from build123d import *

# Parameters (mm, degrees)
BOSS_EXTRUDE1_DEPTH = 0.2
BOSS_EXTRUDE2_DEPTH = 39
CUT_EXTRUDE1_DEPTH  = 10


with BuildPart() as part:
    # Sketch1 → Boss-Extrude1 (new body)
    with BuildSketch(Plane.XY):
        with BuildLine():
            Line((0, 0), (39, 0))
            Line((39, 0), (39, 7.5))
            ThreePointArc((39, 7.5), (37.881966011, 7.763932023), (37, 8.5))
            ThreePointArc((37, 8.5), (35.5, 10), (37, 11.5))
            ThreePointArc((37, 11.5), (37.881966011, 12.236067977), (39, 12.5))
            Line((39, 12.5), (39, 19.5))
            Line((39, 19.5), (0, 19.5))
            Line((0, 19.5), (0, 12.5))
            ThreePointArc((0, 12.5), (1.118033989, 12.236067977), (2, 11.5))
            ThreePointArc((2, 11.5), (3.5, 10), (2, 8.5))
            ThreePointArc((2, 8.5), (1.118033989, 7.763932023), (0, 7.5))
            Line((0, 7.5), (0, 0))
        make_face()
        with BuildLine():
            Line((21, 12.7), (21, 8.9))
            ThreePointArc((21, 8.9), (19.5, 7.4), (18, 8.9))
            Line((18, 8.9), (18, 12.7))
            ThreePointArc((18, 12.7), (19.5, 14.2), (21, 12.7))
        make_face(mode=Mode.SUBTRACT)
    extrude(amount=BOSS_EXTRUDE1_DEPTH)

    # Sketch2 → Boss-Extrude2 (add)
    with BuildSketch(Plane(origin=(39, 0, 0), x_dir=(0, 0, -1), z_dir=(1, 0, 0))):
        with BuildLine():
            Line((-0.7, 0.5), (-0.7, 6.5))
            Line((-0.7, 6.5), (-0.2, 6.5))
            Line((-0.2, 6.5), (-0.2, 0))
            Line((-0.2, 0), (0, 0))
            Line((0, 0), (0, 6.5))
            Line((0, 6.5), (0.5, 6.5))
            Line((0.5, 6.5), (0.5, 0.5))
            ThreePointArc((0.5, 0.5), (-0.1, -0.1), (-0.7, 0.5))
        make_face()
    extrude(amount=-BOSS_EXTRUDE2_DEPTH)

    # Sketch3 → Cut-Extrude1 (cut)
    with BuildSketch(Plane.XY.offset(0.2)):
        Polygon((17, 19.5), (19.5, 17.002927863), (22, 19.5), (22, 22.539691699), (17, 22.539691699), align=None)
    extrude(amount=-CUT_EXTRUDE1_DEPTH, mode=Mode.SUBTRACT)


solid = part.part
Work out the finished part from the listing and answer in its coordinate system (mm). A direction names the side the tool comes from. Give positions to 0.01 mm unless a question says otherwise; leave off trailing zeros. Write each loop counter-clockwise with the first axis right and the second up, starting at its lowest first coordinate (ties: lowest second). Pieces come first, ordered by that corner, then holes.
Q1. Straight lines are drawn through the part: L1, parallel to Z at x = 25, y = 9; L2, parallel to Y at x = 22.5, z = 0.05; L3, parallel to Y at x = 28, z = 0.55. For each, find the intervals that lie inside material, in ascending order.
Answer:
L1: z = 0 to 0.2
L2: y = -0.1 to 19.5
L3: y = 0.1 to 6.5
Q2. The part is cut by section B-B on x = 20.5. Give the vertices of the cut face in (y, z), and give its area (3 significant figures).
Answer:
outline: (0.5, -0.5) - (6.5, -0.5) - (6.5, 0) - (7.78, 0) - (7.78, 0.2) - (6.5, 0.2) - (6.5, 0.7) - (0.5, 0.7) arc R0.6 ccw to start; (13.82, 0) - (18, 0) - (18, 0.2) - (13.82, 0.2) - close
area: 8.86 mm2
Q3. Given pin 1 (2 mm diameter, centred on x = 13, y = 15.5, fed in from -Z); pin 2 (0.5 mm diameter, centred on x = 23.5, z = 0.5, fed in from +Y), each flat-ended and moving along its own axis, determine where each tip first touches the part or whether it passes through.
Answer:
pin 1: stops at z = 0
pin 2: stops at y = 6.5
Q4. The part is cut by section C-C on y = 10. Give the vertices of the cut face in (x, z).
Answer:
outline: (3.5, 0) - (18, 0) - (18, 0.2) - (3.5, 0.2) - close; (21, 0) - (35.5, 0) - (35.5, 0.2) - (21, 0.2) - close
Q5. The part is cut by section D-D on x = 26. Give the vertices of the cut face in (y, z).
Answer:
outline: (0.5, -0.5) - (6.5, -0.5) - (6.5, 0) - (19.5, 0) - (19.5, 0.2) - (6.5, 0.2) - (6.5, 0.7) - (0.5, 0.7) arc R0.6 ccw to start
Q6. The part is cut by section A-A on y = 8. Give the vertices of the cut face in (x, z).
Answer:
outline: (1.5, 0) - (18.3, 0) - (18.3, 0.2) - (1.5, 0.2) - close; (20.7, 0) - (37.5, 0) - (37.5, 0.2) - (20.7, 0.2) - close
Q7. A tool of negligible diameter and unlimited length cuts with its end or side. For faces 1 (the face through (19, 15, 0.2)), 2 (the face through (19, 15, 0)), 3 (the face through (19.8, -0.1, 0.1)), from which of +Z, -Z, +X, -X, +Y, -Y can it reach the whole face along a straight path? Write none if from no direction.
Answer:
face 1: +Z, +X, -X, +Y
face 2: -Z, +X, -X, +Y
face 3: +X, -X, -Y
